Answer from the drawing. Dimensions are ordinates in mm from the lowest x, y and z of the part. A direction names the side the tool comes from. Round coordinates to 2 decimals unless told otherwise and drop trailing zeros. Loops run counter-clockwise (first coordinate to the right, second up) from the corner with the lowest first, then second, coordinate; pieces in that order, holes last.
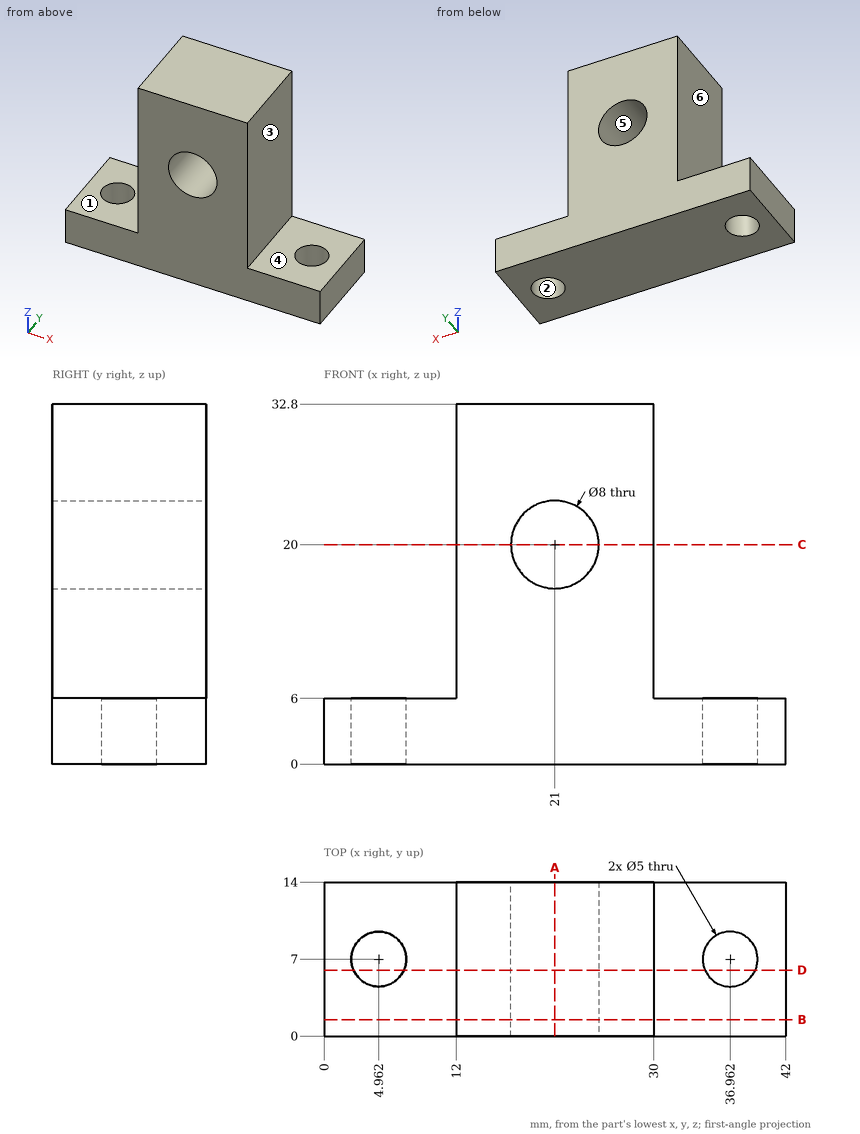
1. Find section A-A (x = 21). Write down the section's boundary in (y, z).
Answer key:
outline: (0, 0) - (14, 0) - (14, 16) - (0, 16) - close; (0, 24) - (14, 24) - (14, 32.8) - (0, 32.8) - close
2. Which of the six approach directions +Z, -Z, +X, -X, +Y, -Y give full straight-line access (tool end or side, diameter ignored) to the marked faces 1, 2 and 3?
Answer key:
face 1: +Z, -X, +Y, -Y
face 2: +Z, -Z
face 3: +Z, +X, +Y, -Y
3. Determine the mould class of the marked faces 4, 5 and 6 for opening direction X: +X half, -X half, draft (parallel to the pull), parting line (faces both ways), or undercut.
Answer key:
face 4: draft
face 5: undercut
face 6: -X half
4. Consider probe 1 along Z at (x, y) = (21, 9.5); probe 2 along Z at (x, y) = (22, 2); probe 3 along X at (y, z) = (5.25, 2). Determine where each line is inside the solid, lowest interval first.
Answer key:
probe 1: z = 0 to 16, 24 to 32.8
probe 2: z = 0 to 16.13, 23.87 to 32.8
probe 3: x = 0 to 3.18, 6.75 to 35.18, 38.75 to 42
5. Find section C-C (z = 20). Write down the section's boundary in (x, y), then the cut area to 3 significant figures.
Answer key:
outline: (12, 0) - (17, 0) - (17, 14) - (12, 14) - close; (25, 0) - (30, 0) - (30, 14) - (25, 14) - close
area: 140 mm2
6. Find section D-D (y = 6). Write down the section's boundary in (x, z).
Answer key:
outline: (0, 0) - (2.67, 0) - (2.67, 6) - (0, 6) - close; (7.25, 0) - (34.67, 0) - (34.67, 6) - (30, 6) - (30, 32.8) - (12, 32.8) - (12, 6) - (7.25, 6) - close; (39.25, 0) - (42, 0) - (42, 6) - (39.25, 6) - close; hole circle Ø8 at (21, 20)
7. Given pin 1 (1.5 mm diameter, centred on y = 10, z = 10, fed in from -X); pin 2 (8 mm diameter, centred on x = 4.96, y = 7, fed in from -Z); pin 3 (3 mm diameter, centred on y = 10, z = 17.5, fed in from +X); pin 4 (8 mm diameter, centred on x = 37.5, z = 21, fed in from -Y), each flat-ended and moving along its own axis, determine where each tip first touches the part or whether it passes through.
Answer key:
pin 1: stops at x = 12
pin 2: stops at z = 0
pin 3: stops at x = 30
pin 4: passes through
8. Find section B-B (y = 1.5). Write down the section's boundary in (x, z), then the cut area to 3 significant figures.
Answer key:
outline: (0, 0) - (42, 0) - (42, 6) - (30, 6) - (30, 32.8) - (12, 32.8) - (12, 6) - (0, 6) - close; hole circle Ø8 at (21, 20)
area: 684 mm2
